```python
from build123d import *

# Parameters (mm, degrees)
ESQUISSE1_R                  = 15
ESQUISSE1_R_2                = 2
BOSS_EXTRU_1_DEPTH           = 4
ENL_V_MAT_EXTRU_1_DEPTH      = 4
R_P_TITION_CIRCULAIRE1_COUNT = 20
ESQUISSE3_R                  = 2
BOSS_EXTRU_2_DEPTH           = 4
ESQUISSE5_R                  = 1.75
BOSS_EXTRU_3_DEPTH           = 2.2
ESQUISSE6_R                  = 4
ENL_V_MAT_EXTRU_2_DEPTH      = 2


with BuildPart() as part:
    # Esquisse1 → Boss.-Extru.1 (new body)
    with BuildSketch(Plane(origin=(0, 0, 0), x_dir=(1, 0, 0), z_dir=(0, 1, 0))):
        with Locations(Location((0, 0, 0), (0, 0, 270))):
            Circle(ESQUISSE1_R)
        with Locations(Location((0, 0, 0), (0, 0, 270))):
            Circle(ESQUISSE1_R_2, mode=Mode.SUBTRACT)
    extrude(amount=BOSS_EXTRU_1_DEPTH)

    # Esquisse2 → Enlèv. mat.-Extru.1 (cut)
    with BuildSketch(Plane(origin=(0, 4, 0), x_dir=(1, 0, 0), z_dir=(0, 1, 0))):
        with BuildLine():
            Line((0.25, 12.5), (-0.25, 12.5))
            add(Edge.make_bspline(
                [(-0.25, 12.5), (-1.210292611, 12.829221626), (-1.046543714, 14.377393022), (-1.981384064, 14.868561369)],
                knots=[0, 0, 0, 0, 1, 1, 1, 1], degree=3))
            ThreePointArc((-1.981384064, 14.868561369), (0, 15.280808024), (1.981384064, 14.868561369))
            add(Edge.make_bspline(
                [(0.25, 12.5), (1.210292611, 12.829221626), (1.046543714, 14.377393022), (1.981384064, 14.868561369)],
                knots=[0, 0, 0, 0, 1, 1, 1, 1], degree=3))
        make_face()
    enl_v_mat_extru_1 = extrude(amount=-ENL_V_MAT_EXTRU_1_DEPTH, mode=Mode.SUBTRACT)

    # Répétition circulaire1: Enlèv. mat.-Extru.1 ×20 about axis
    r_p_tition_circulaire1_axis = Axis((0, 4, 0), (0, 1, 0))
    for i in range(1, R_P_TITION_CIRCULAIRE1_COUNT):
        add(enl_v_mat_extru_1.rotate(r_p_tition_circulaire1_axis, i * 360 / R_P_TITION_CIRCULAIRE1_COUNT), mode=Mode.SUBTRACT)

    # Esquisse3 → Boss.-Extru.2 (add)
    with BuildSketch(Plane(origin=(0, 4, 0), x_dir=(1, 0, 0), z_dir=(0, 1, 0))):
        with BuildLine():
            Line((4, 6.549364769), (4, 30))
            ThreePointArc((4, 30), (0, 34), (-4, 30))
            Line((-4, 30), (-4, 6.549364769))
            Line((-4, 6.549364769), (4, 6.549364769))
        make_face()
        with Locations(Location((0, 30, 0), (0, 0, 270))):
            Circle(ESQUISSE3_R, mode=Mode.SUBTRACT)
    extrude(amount=-BOSS_EXTRU_2_DEPTH)

    # Esquisse5 → Boss.-Extru.3 (add)
    with BuildSketch(Plane(origin=(0, 4, 0), x_dir=(1, 0, 0), z_dir=(0, 1, 0))):
        with Locations(Location((5.9, 0, 0), (0, 0, 270))):
            Circle(ESQUISSE5_R)
        with Locations(Location((0, -5.9, 0), (0, 0, 270))):
            Circle(ESQUISSE5_R)
        with Locations(Location((-5.9, 0, 0), (0, 0, 270))):
            Circle(ESQUISSE5_R)
        with Locations(Location((0, 5.9, 0), (0, 0, 270))):
            Circle(ESQUISSE5_R)
    extrude(amount=BOSS_EXTRU_3_DEPTH)

    # Esquisse6 → Enlèv. mat.-Extru.2 (cut)
    with BuildSketch(Plane(origin=(0, 4, 0), x_dir=(1, 0, 0), z_dir=(0, 1, 0))):
        with Locations(Location((0, 0, 0), (0, 0, 270))):
            Circle(ESQUISSE6_R)
    extrude(amount=-ENL_V_MAT_EXTRU_2_DEPTH, mode=Mode.SUBTRACT)


solid = part.part
```
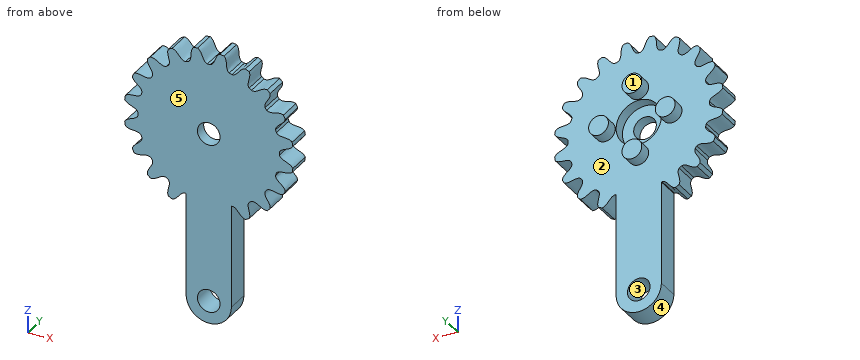
CAD build for the part. Positions are in the model's coordinates, mm. Face numbers are marked on the shaded views. A direction names the side the tool comes from. Coordinates: 2 decimals unless noted, no trailing zeros. Write each loop counter-clockwise with the first axis right and the second up, starting at its lowest first coordinate (ties: lowest second). Pieces come first, ordered by that corner, then holes.
(1) Cut at C-C, the plane y = 0.5. Count the separate pieces of the cut face and the enclosed holes in it, and give its area (3 significant figures).
(2) Cut at A-A, the plane y = 5. List the corners of the cut face in (x, z).
(3) Flat gauge pins, fed straight in: pin 1 (2 mm diameter, centred on y = 3, z = -25.5, fed in from -X); pin 2 (1.5 mm diameter, centred on x = 2, y = 2, fed in from -Z); pin 3 (1 mm diameter, centred on x = 1, y = 1.5, fed in from -Z); pin 4 (2.5 mm diameter, centred on x = 0, z = -30, fed in from -Y). Where does each tip first touch, or does it go through?
(4) Cut at B-B, the plane z = -27.5. List the corners of the cut face in (x, y).
(5) 3-axis set-ups, long thin cutter, end or side, ignore diameter. For the marked faces 1 and 2: which of +Z, -Z, +X, -X, +Y, -Y reach the whole face in a straight line?
(6) Drill centre lines: probe 1 along X at (y, z) = (2.55, -30); probe 2 along X at (y, z) = (3.4, 0); probe 3 along X at (y, z) = (1, -6.5). Where is each one in solid material? Low to high.
(7) Two-plate mould, pull along Z, no slides. Class the marked faces 3, 4 and 5: +Z half, -Z half, draft (parallel to the pull), parting line (faces both ways), or undercut.
Geometry says:
1. separate pieces: 1
1. enclosed holes: 2
1. area: 723 mm2
2. outline: circle Ø3.5 at (-5.9, 0); circle Ø3.5 at (0, -5.9); circle Ø3.5 at (0, 5.9); circle Ø3.5 at (5.9, 0)
3. pin 1: stops at x = -4
3. pin 2: stops at z = -33.8
3. pin 3: stops at z = -33.97
3. pin 4: passes through
4. outline: (-4, 0) - (4, 0) - (4, 4) - (-4, 4) - close
5. face 1: +Z, -Z, +X, -X, +Y
5. face 2: +Y
6. probe 1: x = -4 to -2, 2 to 4
6. probe 2: x = -12.5 to -4, 4 to 12.5
6. probe 3: x = -13.52 to 13.52
7. face 3: undercut
7. face 4: -Z half
7. face 5: draft
